from build123d import *

# Parameters (mm, degrees)
F1_DEPTH = 20
F2_R     = 6.01
F3_DEPTH = 60.001
F5_DEPTH = 7
F6_R     = 4.725935
F6_R_2   = 4.75
F7_DEPTH = 60.001


with BuildPart() as f1:
    # F0 (on Top) → F1 (new body)
    with BuildSketch(Plane.XY):
        with BuildLine():
            Line((-29.436361, 75), (-79.436361, 75))
            ThreePointArc((-79.436361, 75), (-82.971895, 73.535534), (-84.436361, 70))
            Line((-84.436361, 70), (-84.436361, 5))
            ThreePointArc((-84.436361, 5), (-82.971895, 1.464466), (-79.436361, 0))
            Line((-79.436361, 0), (-29.436361, 0))
            ThreePointArc((-29.436361, 0), (-25.900827, 1.464466), (-24.436361, 5))
            Line((-24.436361, 5), (-24.436361, 70))
            ThreePointArc((-24.436361, 70), (-25.900827, 73.535534), (-29.436361, 75))
        make_face()
    extrude(amount=F1_DEPTH)

    # F2 (on face) → F3 (cut, through all)
    with BuildSketch(Plane.YZ.offset(-24.436361)):
        with Locations((60, 20)):
            Circle(F2_R)
        with Locations((15, 20)):
            Circle(F2_R)
    extrude(amount=-F3_DEPTH, mode=Mode.SUBTRACT)

    # F4 (on face) → F5 (join)
    with BuildSketch(Plane.XY.offset(20)):
        Polygon((-55.936361, 53.99), (-54.436361, 53.99), (-52.936361, 53.99), (-52.936361, 66.01), (-55.936361, 66.01), align=None)
        Polygon((-52.936361, 21.01), (-54.436361, 21.01), (-55.936361, 21.01), (-55.936361, 8.828274), (-52.936361, 8.828274), align=None)
    extrude(amount=-F5_DEPTH)

    # F6 (on face) → F7 (cut, through all)
    with BuildSketch(Plane.YZ.offset(-24.436361)):
        with Locations((60, 20)):
            Circle(F6_R)
        with Locations((15, 20)):
            Circle(F6_R_2)
    extrude(amount=-F7_DEPTH, mode=Mode.SUBTRACT)


solid = f1.part
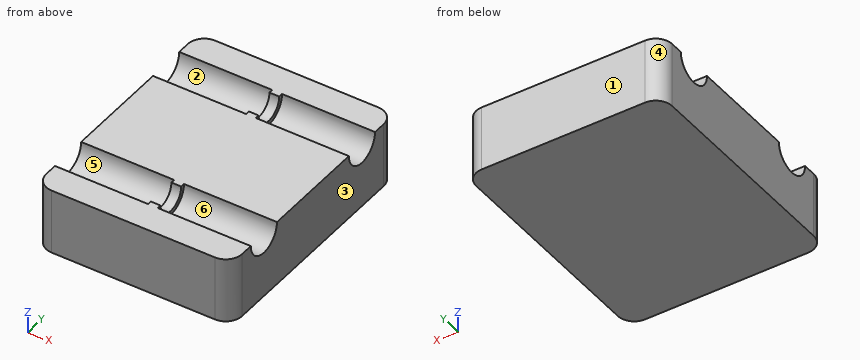
Verification items for the finished model (mm, model axes). Face numbers are marked on the shaded views. A direction names the side the tool comes from. Give positions to 0.01 mm unless a question says otherwise; leave off trailing zeros. Order: outer loops, then holes, each group sorted by start corner. A loop starts at its lowest first (then second) coordinate and runs counter-clockwise, first axis right, second up. Notation, with made-up numbers: M 34.5,40.5 L 44.5,40.5 A20 cw 44.5,66.5 Z; hole C -14,-17.75 d3. An arc over 180 degrees is marked long. Answer as a JSON object with one key per item and string values. Group by question number.
1) Mould release check, pull along Y, two halves, no side actions. Record for the marked faces 1, 2 and 3: released by +Y, released by -Y, zero draft, split by the parting line, or undercut.
2) Scan lines: line 1 along Y through (x, z) = (-46, 18.5); line 2 along Y through (x, z) = (-64.5, 16.75); line 3 along Z through (x, y) = (-62, 14). Record each from-to range of solid material in increasing order. Write a range as [from, to].
3) Access from +Z, -Z, +X, -X, +Y, -Y to the whole of each face (thin tool, end or side, straight path). Record for the marked faces 4, 5 and 6.
4) Depth check by flat-ended pin: pin 1 Ø6 at (x, y) = (-41.5, 32) entering from -Z; pin 2 Ø3 at (y, z) = (16, 18) entering from +X; pin 3 Ø1 at (x, y) = (-52, 57) entering from +Z. Enter the tip coordinate at first touch or a pass-through.
5) Cross-section at C-C (x = -67.5). Enter the section's corners in (y, z), then the cut area to 3 significant figures.
6) Cross-section at B-B (y = 15). Enter the section's corners in (x, z), then the cut area to 3 significant figures.
7) Cross-section at A-A (z = 16.5). Give the number of separate pieces and of enclosed holes in the cut face, then the cut area to 3 significant figures.
Result sheet:
{
 "1": {"face 1": "released by +Y", "face 2": "undercut", "face 3": "zero draft"},
 "2": {"line 1": "y = [0, 9.18], [20.82, 54.18], [65.82, 75]", "line 2": "y = [0, 9.94], [20.06, 54.94], [65.06, 75]", "line 3": "z = [0, 14.07]"},
 "3": {"face 4": "+Z, -Z, -X, +Y", "face 5": "+Z, -X", "face 6": "+Z, +X"},
 "4": {"pin 1": "stops at z = 0", "pin 2": "passes through", "pin 3": "stops at z = 15.11"},
 "5": {"outline": "M 0,0 L 75,0 L 75,20 L 66.01,20 A6.01 cw 53.99,20 L 21.01,20 A6.01 cw 8.99,20 L 0,20 Z", "area": "1,390 mm2"},
 "6": {"outline": "M -84.44,0 L -24.44,0 L -24.44,13.99 L -52.94,13.99 L -52.94,15.25 L -55.94,15.25 L -55.94,13.99 L -84.44,13.99 Z", "area": "843 mm2"},
 "7": {"separate pieces": "3", "enclosed holes": "0", "area": "3,330 mm2"}
}
